Read the model definition and answer for the solid it produces. Units are mm, in the model's axes. Face numbers are marked on the shaded views. A direction names the side the tool comes from. Coordinates: 2 decimals unless noted, no trailing zeros. Loops run counter-clockwise (first coordinate to the right, second up) from the corner with the lowest first, then second, coordinate; pieces in that order, holes last.
from build123d import *

# Parameters (mm, degrees)
F1_DEPTH = 33.02
F2_DEPTH = 48.26
F3_DEPTH = 3.175
F5_DEPTH = 21.591


with BuildPart() as f1:
    # F0 (on Top) → F1 (new body)
    with BuildSketch(Plane.XY):
        with BuildLine():
            Line((0, -17.526), (0, 17.526))
            ThreePointArc((0, 17.526), (-17.526, 0), (0, -17.526))
        make_face()
        with BuildLine():
            ThreePointArc((0, -17.526), (12.3927534471, -12.3927534471), (17.526, 0))
            ThreePointArc((17.526, 0), (12.3927534471, 12.3927534471), (0, 17.526))
            Line((0, 17.526), (0, -17.526))
        make_face()
    extrude(amount=F1_DEPTH)

    # F0 (on Top) → F2 (join)
    with BuildSketch(Plane.XY):
        with BuildLine():
            ThreePointArc((0, -17.526), (12.3927534471, -12.3927534471), (17.526, 0))
            ThreePointArc((17.526, 0), (12.3927534471, 12.3927534471), (0, 17.526))
            Line((0, 17.526), (0, -17.526))
        make_face()
        with BuildLine():
            ThreePointArc((0, 17.526), (12.3927534471, 12.3927534471), (17.526, 0))
            ThreePointArc((17.526, 0), (12.3927534471, -12.3927534471), (0, -17.526))
            Line((0, -17.526), (0, -21.59))
            ThreePointArc((0, -21.59), (15.2664354058, -15.2664354058), (21.59, 0))
            ThreePointArc((21.59, 0), (15.2664354058, 15.2664354058), (0, 21.59))
            Line((0, 21.59), (0, 17.526))
        make_face()
    extrude(amount=-F2_DEPTH)

    # F0 (on Top) → F3 (join)
    with BuildSketch(Plane.XY):
        with BuildLine():
            ThreePointArc((0, -17.526), (-17.526, 0), (0, 17.526))
            Line((0, 17.526), (0, 21.59))
            ThreePointArc((0, 21.59), (-21.59, 0), (0, -21.59))
            Line((0, -21.59), (0, -17.526))
        make_face()
        with BuildLine():
            Line((0, -17.526), (0, 17.526))
            ThreePointArc((0, 17.526), (-17.526, 0), (0, -17.526))
        make_face()
    extrude(amount=-F3_DEPTH)

    # F4 (on face) → F5 (cut, through all)
    with BuildSketch(Plane(origin=(0, 0, 0), x_dir=(0, -1, 0), z_dir=(-1, 0, 0))):
        with BuildLine():
            ThreePointArc((-3.175, -26.67), (0, -29.845), (3.175, -26.67))
            Line((3.175, -26.67), (-3.175, -26.67))
        make_face()
        with BuildLine():
            Line((-3.175, -26.67), (3.175, -26.67))
            ThreePointArc((3.175, -26.67), (0, -23.495), (-3.175, -26.67))
        make_face()
        with BuildLine():
            ThreePointArc((0, -48.26), (-15.2664354058, -41.9364354058), (-21.59, -26.67))
            Line((-21.59, -26.67), (-21.59, -48.26))
            Line((-21.59, -48.26), (0, -48.26))
        make_face()
        with BuildLine():
            Line((21.59, -48.26), (21.59, -26.67))
            ThreePointArc((21.59, -26.67), (15.2664354058, -41.9364354058), (0, -48.26))
            Line((0, -48.26), (21.59, -48.26))
        make_face()
    extrude(amount=-F5_DEPTH, mode=Mode.SUBTRACT)


solid = f1.part
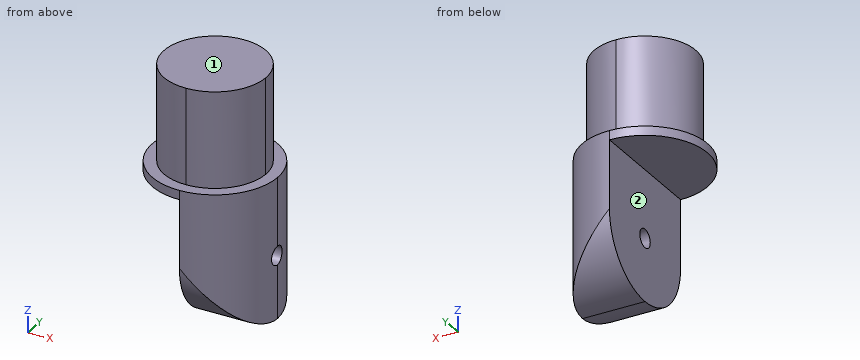
Q1. A cutting plane is placed at A-A (y = -2). Give the vertices of the cut face in (x, z) (1 decimal), then the cut area to 3 significant figures.
Findings below:
outline: (-21.5, -3.2) - (0, -3.2) - (0, -24.2) - (21.5, -24.2) - (21.5, 0) - (17.4, 0) - (17.4, 33) - (-17.4, 33) - (-17.4, 0) - (-21.5, 0) - close; (0, -48.2) - (21.5, -48.2) - (21.5, -29.1) - (0, -29.1) - close
area: 2,150 mm2
Q2. Flat-ended cylindrical pins translate along their axes: pin 1 Ø1.5 at (y, z) = (14, 22) entering from +X; pin 2 Ø1 at (y, z) = (10, 4) entering from -X; pin 3 Ø4 at (y, z) = (16.5, 10) entering from +X; pin 4 Ø5.5 at (y, z) = (0, -26.67) entering from +X. Find the tip coordinate at first contact, or state that the pin passes through.
Findings below:
pin 1: stops at x = 11.47
pin 2: stops at x = -14.73
pin 3: stops at x = 9.84
pin 4: passes through
Q3. A cutting plane is placed at D-D (y = 4). Give the vertices of the cut face in (x, z) (3 decimals), then the cut area to 3 significant figures.
Findings below:
outline: (-21.216, -3.175) - (0, -3.175) - (0, -47.886) - (21.216, -47.886) - (21.216, 0) - (17.063, 0) - (17.063, 33.02) - (-17.063, 33.02) - (-17.063, 0) - (-21.216, 0) - close
area: 2,210 mm2
Q4. Which of the six approach directions +Z, -Z, +X, -X, +Y, -Y give full straight-line access (tool end or side, diameter ignored) to the marked faces 1 and 2?
Findings below:
face 1: +Z, +X, -X, +Y, -Y
face 2: -Z, -X, +Y, -Y
Q5. A cutting plane is placed at B-B (z = 19). Give the vertices of the cut face in (x, y).
Findings below:
outline: circle Ø35.05 at (0, 0)
Q6. Straight lines are drawn through the part: probe 1 along Z at (x, y) = (-9, -6) (3 decimals); probe 2 along Y at (x, z) = (5, -26); probe 3 along Z at (x, y) = (-14.5, 14) (3 decimals). For each, find the intervals that lie inside material, in ascending order.
Findings below:
probe 1: z = -3.175 to 33.02
probe 2: y = -21 to -3.1, 3.1 to 21
probe 3: z = -3.175 to 0
Q7. A cutting plane is placed at C-C (x = -15). Give the vertices of the cut face in (y, z) (3 decimals).
Findings below:
outline: (-15.528, -3.175) - (15.528, -3.175) - (15.528, 0) - (9.064, 0) - (9.064, 33.02) - (-9.064, 33.02) - (-9.064, 0) - (-15.528, 0) - close
